Geometry: final body of the model. Coordinates: model frame, mm. Face numbers are marked on the shaded views. A direction names the side the tool comes from. Give positions to 0.01 mm unless a question says otherwise; leave off trailing zeros. Write each loop counter-clockwise with the first axis right and the second up, starting at its lowest first coordinate (ties: lowest second). Pieces come first, ordered by that corner, then holes.
Q1. Cut plane A-A on y = 20.5. Return the cut outline in (x, z), plus the area to 3 significant figures.
Q2. Reachability of the marked faces 1 and 2 from +Z, -Z, +X, -X, +Y, -Y: full face, straight path, thin tool, end or side. Return the list, or none.
Q3. Pin query (flat end, axial travel): pin 1 (8 mm diameter, centred on x = -7, y = 14, fed in from +Z); pin 2 (2 mm diameter, centred on x = -23.5, z = 32.5, fed in from +Y); pin 3 (1.6 mm diameter, centred on x = -11, z = 1, fed in from -Y). Return the tip coordinate at first contact, or that it passes through.
Q4. Cut plane C-C on x = -13. Return the cut outline in (y, z).
Q5. Cut plane D-D on z = 25. Return the cut outline in (x, y).
Q6. Line query: L1, parallel to X at y = 0.8, z = 11.5; L2, parallel to X at y = 1.1, z = 32.5; L3, parallel to Z at x = -23.5, y = 1.1. Output: solid intervals per line, ascending.
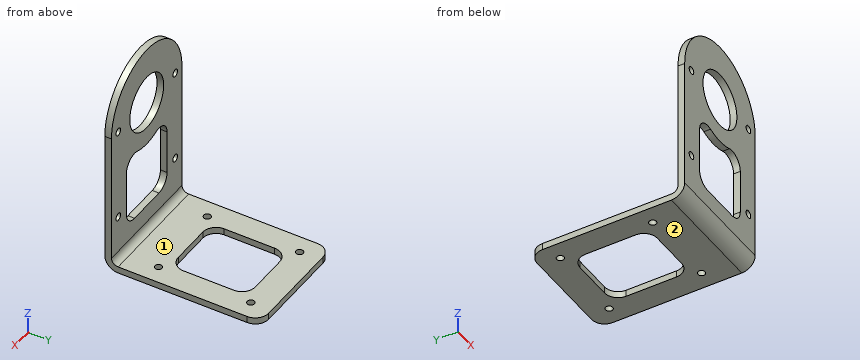
Autodesk Inventor part; units mm, degrees
ref_plane "YZ Plane" through (0, 0, 0) normal (1, 0, 0) x (0, 1, 0)
ref_plane "XZ Plane" through (0, 0, 0) normal (0, 1, 0) x (-1, 0, 0)
ref_plane "XY Plane" through (0, 0, 0) normal (0, 0, 1) x (1, 0, 0)
sketch "スケッチ1" plane through (0, 0, 0) normal (0, 1, 0) x (-1, 0, 0)
  line L0 (26, 0) -> (0, 0)
  line L1 (0, 0) -> (0, -89.5474)
  line L2 (0, -89.5474) -> (26, -89.5474)
  line L3 (26, -89.5474) -> (26, 0)
  line L4 (26, 0) -> (0, 0)
  line L5 (0, 0) -> (0, 70)
  line L6 (0, 70) -> (26, 70)
  line L7 (26, 70) -> (26, 0)
  line L8 (26, 32.5) -> (0, 32.5)
  circle A0 centre (13, 32.5) radius 6.25
  circle A1 centre (13, 32.5) radius 13
  point P0 (26, 32.5)
  point P1 (0, 32.5)
  dimension "d2" = 70
  dimension "d3" = 26
  dimension "d4" = 32.5
  dimension "d5" = 12.5
extrude "プレート1" add sketch "スケッチ1" along normal blind 1.5 contours L0 L5 A1 L7 | A1 L8 A0 | L8 A0 A1
sketch "スケッチ2" plane through (-26, 0, 1.5) normal (0, 0, -1) x (-1, 0, 0)
  line L0 (-26, 0) -> (0, 0)
  line L1 (0, 0) -> (0, 35)
  line L2 (0, 35) -> (-26, 35)
  line L3 (-26, 35) -> (-26, 0)
edge flange "フランジ1" height 35 angle 90 thickness 1.5 bend radius 1.5 thickness toward (0, 0, -1) relief tear relief width 1.5 relief depth 0.75 edges at (-13, 1.5, 0) wall of the first edge with corners at (0, 0, 1.5) (-26, 0, 1.5) (-26, 35, 1.5) (0, 35, 1.5)
bend "曲げ1"
corner "コーナー1"
sketch "スケッチ3" plane through (0, 1.5, 0) normal (0, 1, 0) x (1, 0, 0)
  circle A0 centre (-23.5, -32.5) radius 0.85
  circle A1 centre (-23.5, -11.5) radius 0.85
  circle A2 centre (-2.5, -11.5) radius 0.85
  circle A3 centre (-2.5, -32.5) radius 0.85
  point P0 (0, 0)
extrude "切り取り1" cut sketch "スケッチ3" against normal blind 1.5
sketch "スケッチ4" plane through (0, 35, 0) normal (0, 0, -1) x (-1, 0, 0)
  spline S0 degree 3 poles (4.8, -25.3846) (4.8, -25.2845) (4.78, -25.178) (4.6999, -24.983) (4.6397, -24.8944) (4.4988, -24.7507) (4.4073, -24.6876) (4.208, -24.6046) (4.1004, -24.5846) (3.8988, -24.5846) (3.7907, -24.6049) (3.5913, -24.6885) (3.4999, -24.7517) (3.3597, -24.8953) (3.2999, -24.9835) (3.22, -25.178) (3.2, -25.2844) (3.2, -25.4848) (3.22, -25.5912) (3.2999, -25.7858) (3.3597, -25.8739) (3.4999, -26.0176) (3.5913, -26.0808) (3.7907, -26.1643) (3.8988, -26.1846) (4.1004, -26.1846) (4.208, -26.1646) (4.4073, -26.0816) (4.4988, -26.0186) (4.6397, -25.8748) (4.6999, -25.7862) (4.78, -25.5912) (4.8, -25.4847) (4.8, -25.3846) knots 0 0 0 0 0.060514 0.060514 0.121029 0.121029 0.185215 0.185215 0.249402 0.249402 0.314126 0.314126 0.37885 0.37885 0.439425 0.439425 0.5 0.5 0.560575 0.560575 0.62115 0.62115 0.685874 0.685874 0.750598 0.750598 0.814785 0.814785 0.878971 0.878971 0.939486 0.939486 1 1 1 1
  spline S1 degree 3 poles (4.8, -4.6154) (4.8, -4.5153) (4.78, -4.4088) (4.6999, -4.2138) (4.6397, -4.1252) (4.4988, -3.9814) (4.4073, -3.9184) (4.208, -3.8354) (4.1004, -3.8154) (3.8988, -3.8154) (3.7907, -3.8357) (3.5913, -3.9192) (3.4999, -3.9824) (3.3597, -4.1261) (3.2999, -4.2142) (3.22, -4.4088) (3.2, -4.5152) (3.2, -4.7156) (3.22, -4.822) (3.2999, -5.0165) (3.3597, -5.1047) (3.4999, -5.2483) (3.5913, -5.3115) (3.7907, -5.3951) (3.8988, -5.4154) (4.1004, -5.4154) (4.208, -5.3954) (4.4073, -5.3124) (4.4988, -5.2493) (4.6397, -5.1056) (4.6999, -5.017) (4.78, -4.822) (4.8, -4.7155) (4.8, -4.6154) knots 0 0 0 0 0.060514 0.060514 0.121029 0.121029 0.185215 0.185215 0.249402 0.249402 0.314126 0.314126 0.37885 0.37885 0.439425 0.439425 0.5 0.5 0.560575 0.560575 0.62115 0.62115 0.685874 0.685874 0.750598 0.750598 0.814785 0.814785 0.878971 0.878971 0.939486 0.939486 1 1 1 1
  spline S2 degree 3 poles (22.8, -4.6154) (22.8, -4.5152) (22.78, -4.4088) (22.7001, -4.2142) (22.6403, -4.1261) (22.5001, -3.9824) (22.4087, -3.9192) (22.2093, -3.8357) (22.1012, -3.8154) (21.8996, -3.8154) (21.792, -3.8354) (21.5927, -3.9184) (21.5012, -3.9814) (21.3603, -4.1252) (21.3001, -4.2138) (21.22, -4.4088) (21.2, -4.5153) (21.2, -4.7155) (21.22, -4.822) (21.3001, -5.017) (21.3603, -5.1056) (21.5012, -5.2493) (21.5927, -5.3124) (21.792, -5.3954) (21.8996, -5.4154) (22.1012, -5.4154) (22.2093, -5.3951) (22.4087, -5.3115) (22.5001, -5.2483) (22.6403, -5.1047) (22.7001, -5.0165) (22.78, -4.822) (22.8, -4.7156) (22.8, -4.6154) knots 0 0 0 0 0.060575 0.060575 0.12115 0.12115 0.185874 0.185874 0.250598 0.250598 0.314785 0.314785 0.378971 0.378971 0.439486 0.439486 0.5 0.5 0.560514 0.560514 0.621029 0.621029 0.685215 0.685215 0.749402 0.749402 0.814126 0.814126 0.87885 0.87885 0.939425 0.939425 1 1 1 1
  spline S3 degree 3 poles (22.8, -25.3846) (22.8, -25.2844) (22.78, -25.178) (22.7001, -24.9835) (22.6403, -24.8953) (22.5001, -24.7517) (22.4087, -24.6885) (22.2093, -24.6049) (22.1012, -24.5846) (21.8996, -24.5846) (21.792, -24.6046) (21.5927, -24.6876) (21.5012, -24.7507) (21.3603, -24.8944) (21.3001, -24.983) (21.22, -25.178) (21.2, -25.2845) (21.2, -25.4847) (21.22, -25.5912) (21.3001, -25.7862) (21.3603, -25.8748) (21.5012, -26.0186) (21.5927, -26.0816) (21.792, -26.1646) (21.8996, -26.1846) (22.1012, -26.1846) (22.2093, -26.1643) (22.4087, -26.0808) (22.5001, -26.0176) (22.6403, -25.8739) (22.7001, -25.7858) (22.78, -25.5912) (22.8, -25.4848) (22.8, -25.3846) knots 0 0 0 0 0.060575 0.060575 0.12115 0.12115 0.185874 0.185874 0.250598 0.250598 0.314785 0.314785 0.378971 0.378971 0.439486 0.439486 0.5 0.5 0.560514 0.560514 0.621029 0.621029 0.685215 0.685215 0.749402 0.749402 0.814126 0.814126 0.87885 0.87885 0.939425 0.939425 1 1 1 1
  point P0 (0, -35)
  point P1 (4.8, -25.3846)
  point P2 (4.8, -4.6154)
  point P3 (22.8, -4.6154)
  point P4 (22.8, -25.3846)
extrude "切り取り2" cut sketch "スケッチ4" against normal blind 1.5
sketch "スケッチ5" plane through (0, 1.5, 0) normal (0, 1, 0) x (1, 0, 0)
  line L0 (-20.5, -10) -> (-20.5, -20.0376)
  arc A0 (-20.5, -20.0376) -> (-16.4811, -22.8592) centre (-17.5, -20.0376) ccw
  arc A1 (-9.5189, -22.8592) -> (-16.4811, -22.8592) centre (-13, -32.5) ccw
  arc A2 (-9.5189, -22.8592) -> (-5.5, -20.0376) centre (-8.5, -20.0376) ccw
  line L1 (-5.5, -20.0376) -> (-5.5, -10)
  arc A3 (-5.5, -10) -> (-8.5, -7) centre (-8.5, -10) ccw
  line L2 (-8.5, -7) -> (-17.5, -7)
  arc A4 (-17.5, -7) -> (-20.5, -10) centre (-17.5, -10) ccw
  line L3 (-26, -3) -> (0, -3)
  line L4 (0, -32.5) -> (0, -3)
  arc A5 (-26, -32.5) -> (0, -32.5) centre (-13, -32.5) ccw
  line L5 (-26, -3) -> (-26, -32.5)
  circle A6 centre (-13, -32.5) radius 6.25
  circle A7 centre (-23.5, -32.5) radius 0.85
  circle A8 centre (-2.5, -11.5) radius 0.85
  circle A9 centre (-2.5, -32.5) radius 0.85
  circle A10 centre (-23.5, -11.5) radius 0.85
  point P0 (0, 0)
extrude "切り取り3" cut sketch "スケッチ5" against normal blind 1.5 contours A4 L2 A3 L1 A2 A1 A0 L0
sketch "スケッチ6" plane through (0, 35, 0) normal (0, 0, -1) x (-1, 0, 0)
  line L0 (26, 0) -> (26, -32)
  line L1 (0, 0) -> (26, 0)
  line L2 (0, -32) -> (0, 0)
  circle A0 centre (22, -25.3846) radius 0.8
  circle A1 centre (4, -25.3846) radius 0.8
  circle A2 centre (4, -4.6154) radius 0.8
  circle A3 centre (22, -4.6154) radius 0.8
  line L3 (22, -25.3846) -> (4, -4.6154)
  line L4 (4, -25.3846) -> (22, -4.6154)
  line L5 (17.5, -23.6538) -> (8.5, -23.6538)
  line L6 (5.5, -20.6538) -> (5.5, -9.3462)
  line L7 (8.5, -6.3462) -> (17.5, -6.3462)
  line L8 (20.5, -9.3462) -> (20.5, -20.6538)
  arc A4 (26, -3) -> (23, 0) centre (23, -3) ccw
  line L9 (0, 0) -> (26, 0)
  arc A5 (3, 0) -> (0, -3) centre (3, -3) ccw
  arc A6 (17.5, -23.6538) -> (20.5, -20.6538) centre (17.5, -20.6538) ccw
  arc A7 (5.5, -20.6538) -> (8.5, -23.6538) centre (8.5, -20.6538) ccw
  arc A8 (8.5, -6.3462) -> (5.5, -9.3462) centre (8.5, -9.3462) ccw
  arc A9 (20.5, -9.3462) -> (17.5, -6.3462) centre (17.5, -9.3462) ccw
  point P0 (0, -35)
  point P1 (20.5, -23.6538)
  point P2 (5.5, -6.3462)
  point P3 (5.5, -23.6538)
  dimension "d29" = 1.5
  dimension "d30" = 3
  dimension "d31" = 3
  dimension "d32" = 3
extrude "切り取り4" cut sketch "スケッチ6" against normal blind 1.5 contours L0 A4 L1 | L1 A5 L2 | A6 L5 A7 L4 L3 | L3 L4 A9 L8 A6 | L4 A7 L6 A8 L3 | L3 A8 L7 A9 L4
equation "\"d23\" = Thickness"
equation "\"d25\" = Thickness"
equation "\"d27\" = Thickness"
equation "\"d33\" = Thickness"
equation "\"d12\" = Thickness"
equation "\"d13\" = BendReliefWidth"
equation "\"d14\" = BendReliefDepth"
equation "\"d15\" = MinimumRemnant"
equation "\"d16\" = TransitionRadius"
equation "\"d19\" = BendRadius"
equation "\"d20\" = CornerReliefSize"
equation "\"d21\" = GapSize"
equation "\"d22\" = JacobiRadiusSize"
equation "\"BendRadius\" = Thickness"
equation "\"BendReliefWidth\" = Thickness"
equation "\"BendReliefDepth\" = 0.5 * Thickness"
equation "\"CornerReliefSize\" = 4 * Thickness"
equation "\"MinimumRemnant\" = 2 * Thickness"
equation "\"TransitionRadius\" = BendRadius"
equation "\"JacobiRadiusSize\" = BendRadius"
equation "\"GapSize\" = Thickness"
properties part number "toe_back" material "アルミニウム 6061"
Data:
1. outline: (-26, 0) - (-20.5, 0) - (-20.5, 1.5) - (-26, 1.5) - close; (-5.5, 0) - (0, 0) - (0, 1.5) - (-5.5, 1.5) - close
1. area: 16.5 mm2
2. face 1: +Z, +X, -X, +Y
2. face 2: -Z, +X, -X, +Y, -Y
3. pin 1: stops at z = 1.5
3. pin 2: stops at y = 1.5
3. pin 3: stops at y = 0.25
4. outline: (0, 3) arc R3 ccw to (3, 0) - (11.35, 0) - (11.35, 1.5) - (3, 1.5) arc R1.5 cw to (1.5, 3) - (1.5, 7) - (0, 7) - close; (0, 22.25) - (1.5, 22.25) - (1.5, 26.25) - (0, 26.25) - close; (0, 38.75) - (1.5, 38.75) - (1.5, 45.5) - (0, 45.5) - close; (28.65, 0) - (35, 0) - (35, 1.5) - (28.65, 1.5) - close
5. outline: (-26, 0) - (0, 0) - (0, 1.5) - (-26, 1.5) - close
6. L1: x = -26 to -24.35, -22.65 to -20.5, -5.5 to -3.35, -1.65 to 0
6. L2: x = -26 to -24.35, -22.65 to -19.25, -6.75 to -3.35, -1.65 to 0
6. L3: z = 0.68 to 10.65, 12.35 to 31.65, 33.35 to 40.16
